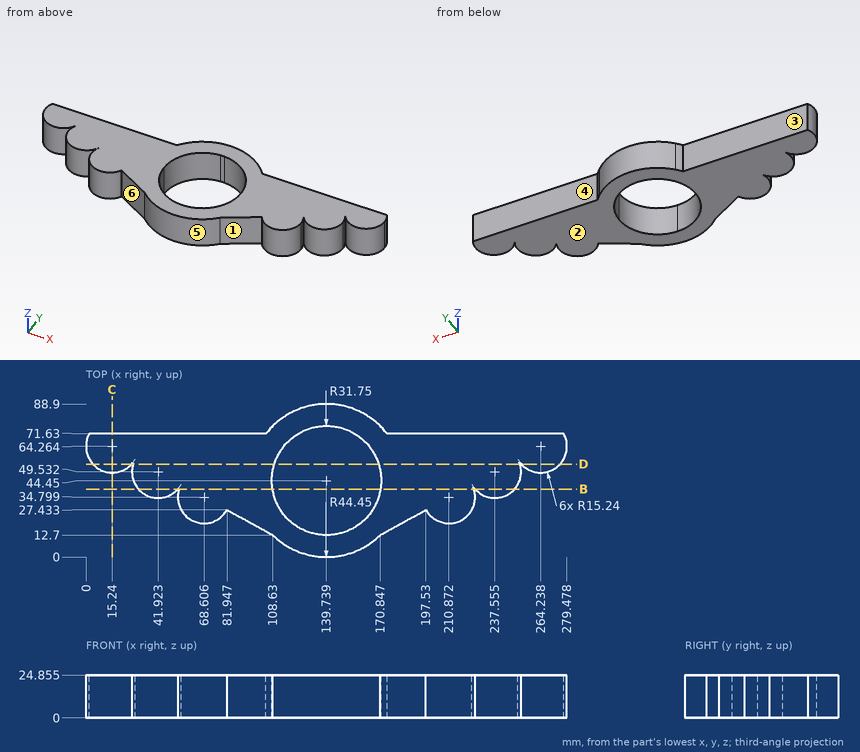
Study the drawing (mm; zero at the part's minimum x, y, z) and answer. A direction names the side the tool comes from. Give positions to 0.01 mm unless a question says otherwise; leave off trailing zeros. Write each loop counter-clockwise with the first axis right and the second up, starting at its lowest first coordinate (ties: lowest second). Pieces come first, ordered by that corner, then holes. Notation, with made-up numbers: (73.5, -15) - (87.5, -15) arc R12 ccw to (87.5, -3) - close; hole circle Ø6 at (68, 30). An arc over 180 degrees is marked (long way). One line per question, with ' | ' between items. Start each with the question number.
1. Section C-C, the plane x = 15.24 is taken. Determine the outline of the cut face in (y, z) (1 decimal).
2. Straight lines are drawn through the part: line 1 (X direction, y = 59, z = 6.75); line 2 (Y direction, x = 15.5, z = 8); line 3 (X direction, y = 59.5, z = 6.5) (1 decimal). For each, find the intervals that lie inside material, in ascending order.
3. Section B-B, the plane y = 39.5 is taken. Count the separate pieces of the cut face and the enclosed holes in it, then the cut area to 3 significant figures.
4. For the marked faces 1, 2 and 3, determine the directions among +Z, -Z, +X, -X, +Y, -Y from which every point of the face is accessible in a straight line to the end or side of a thin tool.
5. Given P1, Ø8, axis at y = 55, z = 21, coming from the -X side; P2, Ø1, axis at x = 137, z = 4, coming from the -Y side; P3, Ø3, axis at y = 11.5, z = 8.5, coming from the +X side, each flat-ended and moving along its own axis, determine where each tip first touches the part or whether it passes through.
6. Section D-D, the plane y = 54 is taken. Determine the outline of the cut face in (x, z) (1 decimal), then the cut area to 3 significant figures.
7. Determine the mould class of the marked faces 4, 5 and 6 for opening direction X: +X half, -X half, draft (parallel to the pull), parting line (faces both ways), or undercut.
Result:
1) outline: (49, 0) - (71.6, 0) - (71.6, 24.9) - (49, 24.9) - close
2) line 1: x = 0.94 to 111.52, 167.96 to 278.54 | line 2: y = 49.03 to 71.63 | line 3: x = 0.8 to 111.8, 167.7 to 278.7
3) separate pieces: 4 | enclosed holes: 0 | area: 3,840 mm2
4) face 1: +Z, -Z, -Y | face 2: -Z, +X, -X, +Y, -Y | face 3: +Z, -Z, -X, +Y
5) P1: stops at x = 0.94 | P2: stops at y = 0.06 | P3: stops at x = 171.39
6) outline: (4, 0) - (26.5, 0) - (26.5, 24.9) - (4, 24.9) - close; (27.4, 0) - (109.5, 0) - (109.5, 24.9) - (27.4, 24.9) - close; (170, 0) - (252.1, 0) - (252.1, 24.9) - (170, 24.9) - close; (253, 0) - (275.5, 0) - (275.5, 24.9) - (253, 24.9) - close | area: 5,200 mm2
7) face 4: draft | face 5: parting line | face 6: undercut
